```python
from build123d import *

# Parameters (mm, degrees)
PAD_DEPTH       = 5
SKETCH001_W     = 10
SKETCH001_H     = 21
PAD001_DEPTH    = 54
PAD002_DEPTH    = 5
SKETCH004_W     = 5
SKETCH004_H     = 12
PAD003_DEPTH    = 40
SKETCH005_W     = 10
SKETCH005_H     = 21
PAD004_DEPTH    = 25.5
PAD005_DEPTH    = 10
SKETCH007_R     = 2.5
POCKET_DEPTH    = 10
SKETCH008_R     = 10.5
SKETCH008_R_2   = 7.5
PAD006_DEPTH    = 30
CHAMFER_SIZE    = 4
FILLET_R        = 4
FILLET001_R     = 4
FILLET002_R     = 4
SKETCH009_W     = 3
SKETCH009_H     = 20
POCKET001_DEPTH = 10
SKETCH010_R     = 7.5
PAD007_DEPTH    = 5
FILLET003_R     = 4
FILLET004_R     = 4
PAD008_DEPTH    = 10
SKETCH012_W     = 74
SKETCH012_H     = 4
SKETCH012_W_2   = 10
SKETCH012_H_2   = 8
PAD009_DEPTH    = 2
FILLET005_R     = 7
FILLET006_R     = 7
FILLET007_R     = 3
FILLET008_R     = 2
FILLET009_R     = 3
FILLET010_R     = 1
FILLET011_R     = 1
FILLET012_R     = 1


with BuildPart() as part:
    # Sketch → Pad (new body)
    with BuildSketch(Plane.XY):
        with BuildLine():
            Line((0, 21), (0, 0))
            Line((0, 0), (10, 0))
            Line((136.5, 0), (10, 0))
            Line((141.5, 0), (136.5, 0))
            ThreePointArc((141.5, 0), (135.349242, 14.849242), (120.5, 21))
            Line((10, 21), (120.5, 21))
            Line((0, 21), (10, 21))
        make_face()
    extrude(amount=PAD_DEPTH)

    # Sketch001 (on Face4 of Pad) → Pad001 (join)
    with BuildSketch(Plane.XY.offset(5)):
        with Locations((5, 10.5)):
            Rectangle(SKETCH001_W, SKETCH001_H)
    extrude(amount=PAD001_DEPTH)

    # Sketch002 (on Face3 of Pad001) → Pad002 (join)
    with BuildSketch(Plane.XY.offset(5)):
        with BuildLine():
            ThreePointArc((136.5, 0), (131.813708, 11.313708), (120.5, 16))
            Line((120.5, 16), (120.5, 21))
            ThreePointArc((141.5, 0), (135.349242, 14.849242), (120.5, 21))
            Line((136.5, 0), (141.5, 0))
        make_face()
    extrude(amount=PAD002_DEPTH)

    # Sketch004 (on Face5 of Pad002) → Pad003 (join)
    with BuildSketch(Plane.YZ.offset(10)):
        with Locations((18.5, 53)):
            Rectangle(SKETCH004_W, SKETCH004_H)
    extrude(amount=PAD003_DEPTH)

    # Sketch005 (on Face14 of Pad003) → Pad004 (join)
    with BuildSketch(Plane.XY.offset(59)):
        with Locations((5, 10.5)):
            Rectangle(SKETCH005_W, SKETCH005_H)
    extrude(amount=PAD004_DEPTH)

    # Sketch006 (on Face1 of Pad004) → Pad005 (join)
    with BuildSketch(Plane.XY.offset(84.5)):
        Polygon((0, 0), (31, 0), (31, 21), (10, 21), (0, 21), align=None)
    extrude(amount=PAD005_DEPTH)

    # Sketch007 (on Face11 of Pad005) → Pocket (cut)
    with BuildSketch(Plane.XY.offset(94.5)):
        with Locations((20.5, 10.5)):
            Circle(SKETCH007_R)
    extrude(amount=-POCKET_DEPTH, mode=Mode.SUBTRACT)

    # Sketch008 (on Face10 of Pocket) → Pad006 (join)
    with BuildSketch(Plane.XY.offset(94.5)):
        with Locations((20.5, 10.5)):
            Circle(SKETCH008_R)
        with Locations((20.5, 10.5)):
            Circle(SKETCH008_R_2, mode=Mode.SUBTRACT)
    extrude(amount=PAD006_DEPTH)

    # Chamfer
    chamfer_edges = [part.edges().sort_by_distance(p)[0] for p in [
        (135.349242, 14.849242, 10),
    ]]
    chamfer(chamfer_edges, length=CHAMFER_SIZE)

    # Fillet
    fillet_edges = [part.edges().sort_by_distance(p)[0] for p in [
        (50, 21, 53),
    ]]
    fillet(fillet_edges, radius=FILLET_R)

    # Fillet001
    fillet001_edges = [part.edges().sort_by_distance(p)[0] for p in [
        (0, 10.5, 0),
    ]]
    fillet(fillet001_edges, radius=FILLET001_R)

    # Fillet002
    fillet002_edges = [part.edges().sort_by_distance(p)[0] for p in [
        (0, 21, 49.25),
    ]]
    fillet(fillet002_edges, radius=FILLET002_R)

    # Sketch009 (on Face6 of Fillet002) → Pocket001 (cut)
    with BuildSketch(Plane.YZ.offset(10)):
        with Locations((1.5, 37)):
            Rectangle(SKETCH009_W, SKETCH009_H)
    extrude(amount=-POCKET001_DEPTH, mode=Mode.SUBTRACT)

    # Sketch010 (on Face33 of Pocket001) → Pad007 (join)
    with BuildSketch(Plane.XY.offset(124.5)):
        Polygon((-11.5, -10), (52.5, -10), (62.5, -10), (62.5, 21), (52.5, 21), (-11.5, 21), align=None)
        with Locations((20.5, 10.5)):
            Circle(SKETCH010_R, mode=Mode.SUBTRACT)
    extrude(amount=PAD007_DEPTH)

    # Fillet003
    fillet003_edges = [part.edges().sort_by_distance(p)[0] for p in [
        (0, 8.5, 94.5),
    ]]
    fillet(fillet003_edges, radius=FILLET003_R)

    # Fillet004
    fillet004_edges = [part.edges().sort_by_distance(p)[0] for p in [
        (28, 21, 47),
    ]]
    fillet(fillet004_edges, radius=FILLET004_R)

    # Sketch011 (on Face43 of Fillet004) → Pad008 (join)
    with BuildSketch(Plane.XZ.offset(10)):
        Polygon((62.5, 163.5), (-16, 157.177852), (-12, 149.5), (-12, 153.5), (52.5, 153.5), (52.5, 129.5), (62.5, 129.5), (62.5, 153.5), align=None)
    extrude(amount=-PAD008_DEPTH)

    # Sketch012 (on Face45 of Pad008) → Pad009 (join)
    with BuildSketch(Plane(origin=(0, 0, 0), x_dir=(-1, 0, 0), z_dir=(0, 1, 0))):
        with Locations((-25.5, 131.5)):
            Rectangle(SKETCH012_W, SKETCH012_H)
        with Locations((-20.25, 153.5)):
            Rectangle(SKETCH012_W_2, SKETCH012_H_2)
    extrude(amount=PAD009_DEPTH)

    # Fillet005
    fillet005_edges = [part.edges().sort_by_distance(p)[0] for p in [
        (-11.5, 21, 127),
    ]]
    fillet(fillet005_edges, radius=FILLET005_R)

    # Fillet006
    fillet006_edges = [part.edges().sort_by_distance(p)[0] for p in [
        (62.5, 21, 127),
    ]]
    fillet(fillet006_edges, radius=FILLET006_R)

    # Fillet007
    fillet007_edges = [part.edges().sort_by_distance(p)[0] for p in [
        (62.5, -5, 163.5),
    ]]
    fillet(fillet007_edges, radius=FILLET007_R)

    # Fillet008
    fillet008_edges = [part.edges().sort_by_distance(p)[0] for p in [
        (-16, -5, 157.177852),
    ]]
    fillet(fillet008_edges, radius=FILLET008_R)

    # Fillet009
    fillet009_edges = [part.edges().sort_by_distance(p)[0] for p in [
        (-11.5, -10, 127),
    ]]
    fillet(fillet009_edges, radius=FILLET009_R)

    # Fillet010
    fillet010_edges = [part.edges().sort_by_distance(p)[0] for p in [
        (20.25, 2, 157.5),
    ]]
    fillet(fillet010_edges, radius=FILLET010_R)

    # Fillet011
    fillet011_edges = [part.edges().sort_by_distance(p)[0] for p in [
        (15.25, 2, 153),
    ]]
    fillet(fillet011_edges, radius=FILLET011_R)

    # Fillet012
    fillet012_edges = [part.edges().sort_by_distance(p)[0] for p in [
        (25.25, 2, 153),
    ]]
    fillet(fillet012_edges, radius=FILLET012_R)


solid = part.part
```
Input: part model. Units: mm. Frame: model coordinates. A direction names the side the tool comes from. Give positions to 0.01 mm unless a question says otherwise; leave off trailing zeros. Order: outer loops, then holes, each group sorted by start corner. A loop starts at its lowest first (then second) coordinate and runs counter-clockwise, first axis right, second up. Notation, with made-up numbers: (78.5, 70) - (134.5, 70) arc R18 cw to (134.5, 82) - close; hole circle Ø1 at (47.25, 56.25). An arc over 180 degrees is marked (long way). Put each result on its own line as item: value.
Item 1: Section query C-C, the plane z = 75. Return loops of the section in (x, y), then the cut area to 3 significant figures.
Found:
outline: (0, 0) - (10, 0) - (10, 21) - (4, 21) arc R4 ccw to (0, 17) - close
area: 207 mm^2
Item 2: Contact query for flat-ended pins moving along their axis: pin 1 (5 mm diameter, centred on x = 18.5, y = -3, fed in from +Z); pin 2 (8 mm diameter, centred on y = -4.5, z = 139, fed in from -X); pin 3 (6 mm diameter, centred on x = 24.5, z = 50.5, fed in from -Y). Output: stop coordinate, or through.
Found:
pin 1: stops at z = 160.16
pin 2: stops at x = 52.5
pin 3: stops at y = 16
Item 3: Section query D-D, the plane x = 111.5. Return loops of the section in (y, z).
Found:
outline: (0, 0) - (17, 0) arc R4 ccw to (21, 4) - (21, 5) - (0, 5) - close
Item 4: Section query B-B, the plane x = 34. Return loops of the section in (y, z), then the cut area to 3 significant figures.
Found:
outline: (-10, 124.5) - (21, 124.5) - (21, 129.5) - (2, 129.5) - (2, 133.5) - (0, 133.5) - (0, 129.5) - (-10, 129.5) - close; (-10, 153.5) - (0, 153.5) - (0, 161.2) - (-10, 161.2) - close; (0, 0) - (17, 0) arc R4 ccw to (21, 4) - (21, 5) - (0, 5) - close; (16, 47) - (17, 47) arc R4 ccw to (21, 51) - (21, 59) - (16, 59) - close
area: 398 mm^2
Item 5: Access query for faces 4 (the flat face through (30, 16, 53)), 5 (the cylindrical face through (10.3, 20.25, 92.83)), 6 (the flat face through (62.5, -4, 138)). Directions: +Z, -Z, +X, -X, +Y, -Y. A direction counts if a zero-diameter tool reaches every point of the face in a straight line with its end or side. Return the directions, or none.
Found:
face 4: +X, -Y
face 5: -X, +Y
face 6: +Z, +X, +Y, -Y
Item 6: Draft query along X for faces 1 (the cylindrical face through (1.203, 8.381, 93.359)), 2 (the flat face through (5, 3, 37)), 3 (the flat face through (24, 11, 94.5)). Return one class per face: +X half, -X half, draft (parallel to the pull), parting line (faces both ways), or undercut.
Found:
face 1: -X half
face 2: draft
face 3: undercut
Item 7: Section query A-A, the plane z = 127. Return loops of the section in (x, y).
Found:
outline: (-11.5, -7) arc R3 ccw to (-8.5, -10) - (62.5, -10) - (62.5, 14) arc R7 ccw to (55.5, 21) - (-4.5, 21) arc R7 ccw to (-11.5, 14) - close; hole circle Ø15 at (20.5, 10.5)
Item 8: Ray query, L1, parallel to Y at x = 20, z = 102; L2, parallel to Z at x = 38.5, y = 5.5; L3, parallel to Y at x = 20.5, z = 87.75. Return the intervals inside material, ascending. Write a range as from..to.
Found:
L1: y = 0.01..3.02, 17.98..20.99
L2: z = 0..5, 124.5..129.5
L3: y = 0..8, 13..21
